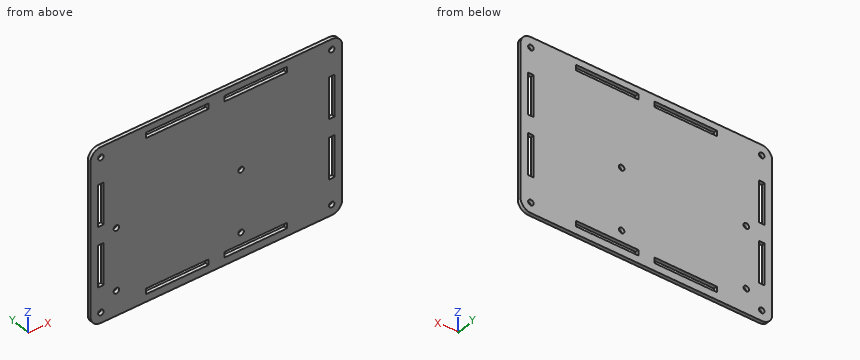
from build123d import *

# Parameters (mm, degrees)
SKETCH1_W           = 145.34
SKETCH1_H           = 100.51
SKETCH1_R           = 1.6
SKETCH1_W_2         = 36
SKETCH1_H_2         = 3.2
SKETCH1_W_3         = 3.2
SKETCH1_H_3         = 24
BOSS_EXTRUDE1_DEPTH = 2
FILLET1_R           = 6
FILLET2_R           = 6
FILLET3_R           = 6


with BuildPart() as part:
    # Sketch1 → Boss-Extrude1 (new body)
    with BuildSketch(Plane(origin=(0, 0, 0), x_dir=(1, 0, 0), z_dir=(0, 1, 0))):
        with Locations((72.67, 50.255)):
            Rectangle(SKETCH1_W, SKETCH1_H)
        with Locations(Location((14.946, 86.224, 0), (0, 0, 270))):
            Circle(SKETCH1_R, mode=Mode.SUBTRACT)
        with Locations(Location((86.952, 86.224, 0), (0, 0, 270))):
            Circle(SKETCH1_R, mode=Mode.SUBTRACT)
        with Locations(Location((86.952, 50.413, 0), (0, 0, 270))):
            Circle(SKETCH1_R, mode=Mode.SUBTRACT)
        with Locations(Location((14.946, 50.413, 0), (0, 0, 270))):
            Circle(SKETCH1_R, mode=Mode.SUBTRACT)
        with Locations(Location((6, 94.51, 0), (0, 0, 270))):
            Circle(SKETCH1_R, mode=Mode.SUBTRACT)
        with Locations(Location((139.34, 94.51, 0), (0, 0, 270))):
            Circle(SKETCH1_R, mode=Mode.SUBTRACT)
        with Locations(Location((139.34, 6, 0), (0, 0, 270))):
            Circle(SKETCH1_R, mode=Mode.SUBTRACT)
        with Locations(Location((6, 6, 0), (0, 0, 270))):
            Circle(SKETCH1_R, mode=Mode.SUBTRACT)
        with Locations((50, 5.414130674)):
            Rectangle(SKETCH1_W_2, SKETCH1_H_2, mode=Mode.SUBTRACT)
        with Locations((50, 94.51)):
            Rectangle(SKETCH1_W_2, SKETCH1_H_2, mode=Mode.SUBTRACT)
        with Locations((95.34, 94.51)):
            Rectangle(SKETCH1_W_2, SKETCH1_H_2, mode=Mode.SUBTRACT)
        with Locations((95.34, 5.414130674)):
            Rectangle(SKETCH1_W_2, SKETCH1_H_2, mode=Mode.SUBTRACT)
        with Locations((6, 67.51)):
            Rectangle(SKETCH1_W_3, SKETCH1_H_3, mode=Mode.SUBTRACT)
        with Locations((6, 33)):
            Rectangle(SKETCH1_W_3, SKETCH1_H_3, mode=Mode.SUBTRACT)
        with Locations((139.34, 67.51)):
            Rectangle(SKETCH1_W_3, SKETCH1_H_3, mode=Mode.SUBTRACT)
        with Locations((139.34, 33)):
            Rectangle(SKETCH1_W_3, SKETCH1_H_3, mode=Mode.SUBTRACT)
    extrude(amount=BOSS_EXTRUDE1_DEPTH)

    # Fillet1
    fillet1_edges = [part.edges().sort_by_distance(p)[0] for p in [
        (0, 1, -100.51),
    ]]
    fillet(fillet1_edges, radius=FILLET1_R)

    # Fillet2
    fillet2_edges = [part.edges().sort_by_distance(p)[0] for p in [
        (0, 1, 0),
    ]]
    fillet(fillet2_edges, radius=FILLET2_R)

    # Fillet3
    fillet3_edges = [part.edges().sort_by_distance(p)[0] for p in [
        (145.34, 1, -100.51),
        (145.34, 1, 0),
    ]]
    fillet(fillet3_edges, radius=FILLET3_R)


solid = part.part
Design review of the part built by this model. Coordinates are the model's own, in mm. Coordinates: 2 decimals unless noted, no trailing zeros. Order: outer loops, then holes, each group sorted by start corner. A loop starts at its lowest first (then second) coordinate and runs counter-clockwise, first axis right, second up. Notation, with made-up numbers: (37.25, 27.5) -> (60.25, 27.5) arc R12 cw to (60.25, 48.5) -> close; hole circle Ø6 at (-18, -15.75). An arc over 180 degrees is marked (long way). Use one line per item in the form item = value. Start each with the question number.
(1) Add section C-C on y = 1.65. Give the number of separate pieces and of enclosed holes in the cut face, plus the area to 3 significant figures.
(2) Add section B-B on z = -31. State the section outline as (x, y) points.
(3) For probe 1 along Z at (x, y) = (112.5, 0.3); probe 2 along Z at (x, y) = (139.5, 1.05); probe 3 along X at (y, z) = (1.2, -94.51), list the stretches that pass through material, from the lowest coordinate up.
(4) Add section A-A on x = 49. State the section outline as (y, z) points.
(5) Insertion check: pin 1 (2.5 mm diameter, centred on x = 86.952, z = -86.224, fed in from -Y); pin 2 (0.6 mm diameter, centred on y = 1, z = -5.5, fed in from -X); pin 3 (0.6 mm diameter, centred on y = 0.5, z = -4.5, fed in from +X); pin 4 (0.6 mm diameter, centred on x = 140, y = 0.5, fed in from +Z). Each pin has a flat end and moves straight along its axis. Give the tip position at first contact, or say it passes through.
Answer block:
q1.separate_pieces = 1
q1.enclosed_holes = 16
q1.area = 13,700 mm²
q2.outline = (0, 0) -> (4.4, 0) -> (4.4, 2) -> (0, 2) -> close; (7.6, 0) -> (137.74, 0) -> (137.74, 2) -> (7.6, 2) -> close; (140.94, 0) -> (145.34, 0) -> (145.34, 2) -> (140.94, 2) -> close
q3.probe_1 = -100.51 to -96.11, -92.91 to -7.01, -3.81 to 0
q3.probe_2 = -100.51 to -96.1, -92.92 to -79.51, -55.51 to -45, -21 to -7.59, -4.41 to 0
q3.probe_3 = 0 to 4.4, 7.6 to 32, 68 to 77.34, 113.34 to 137.74, 140.94 to 145.34
q4.outline = (0, -100.51) -> (2, -100.51) -> (2, -96.11) -> (0, -96.11) -> close; (0, -92.91) -> (2, -92.91) -> (2, -7.01) -> (0, -7.01) -> close; (0, -3.81) -> (2, -3.81) -> (2, 0) -> (0, 0) -> close
q5.pin_1 = through
q5.pin_2 = 0
q5.pin_3 = 145.22
q5.pin_4 = -0.01
